```python
from build123d import *


# Read off the part's stored shape, not the designer's step: Shell1
with BuildPart() as part:
    # Sketch3 → Revolve1 (revolve)
    with BuildSketch(Plane(origin=(0, 0, 0), x_dir=(0, 0, -1), z_dir=(1, 0, 0)), mode=Mode.PRIVATE) as revolve1_sk:
        Polygon((-144.855352602, 25), (5.144647398, 25), (5.144647398, 22), (6.144647398, 22), (26.144647398, 20.250226729), (26.144647398, 0), (-144.855352602, 0), align=None)
    revolve(revolve1_sk.sketch.rotate(Axis((0, 0, 32.959641256), (0, 0, -1)), 90), axis=Axis((0, 0, 32.959641256), (0, 0, -1)))

    # Shell1 outline → Shell1 (revolve, cut)
    with BuildSketch(Plane.XZ):
        Polygon((19, -2.144647398), (22, -2.144647398), (22, 144.855352602), (0, 144.855352602), (0, -26.144647398), (17.238767217, -26.144647398), (19, -6.013664569), align=None)
    revolve(axis=Axis((0, 0, 0), (0, 0, 1)), mode=Mode.SUBTRACT)

    # Sketch4 → Revolve3 (revolve)
    with BuildSketch(Plane(origin=(0, 0, 0), x_dir=(0, 0, -1), z_dir=(1, 0, 0)), mode=Mode.PRIVATE) as revolve3_sk:
        with BuildLine():
            Line((-15.655352602, 37.557879022), (-15.655352602, 25))
            Line((-15.655352602, 25), (5.144647398, 25))
            Line((5.144647398, 25), (5.144647398, 37.557879022))
            Line((5.144647398, 37.557879022), (0.144647398, 37.557879022))
            ThreePointArc((0.144647398, 37.557879022), (-2.092417968, 32.142324694), (-2.855352602, 26.332796239))
            Line((-2.855352602, 26.332796239), (-7.655352602, 26.332796239))
            ThreePointArc((-7.655352602, 26.332796239), (-8.418287237, 32.142324694), (-10.655352602, 37.557879022))
            Line((-10.655352602, 37.557879022), (-15.655352602, 37.557879022))
        make_face()
    revolve(revolve3_sk.sketch.rotate(Axis((0, 0, -29.694647398), (0, 0, 1)), 90), axis=Axis((0, 0, -29.694647398), (0, 0, 1)))


solid = part.part
```
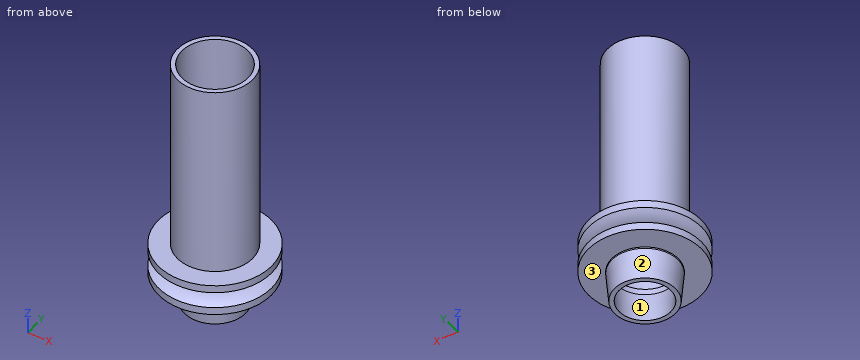
Here's how the part is built. I have some questions about the finished solid (model axes, mm). Face numbers are marked on the shaded views. Coordinates: 2 decimals unless noted, no trailing zeros. Write each loop counter-clockwise with the first axis right and the second up, starting at its lowest first coordinate (ties: lowest second). Pieces come first, ordered by that corner, then holes. Notation, with made-up numbers: (77, 43) -> (111, 43) arc R11 ccw to (111, 59) -> close; hole circle Ø10 at (10.5, 88.25). An arc over 180 degrees is marked (long way). Use a Markdown table: item, result. Add a question column.
(1) I'm going to push flat-ended pins straight in: P1, Ø5, axis at x = -13.5, z = 64.5, coming from the -Y side; P2, Ø12, axis at x = 8.5, z = 78, coming from the -Y side; P3, Ø10, axis at x = -4.5, z = 85.5, coming from the -Y side; P4, Ø22.5, axis at x = -11, y = 3.5, coming from the -Z side. Where does each tip first touch, or does it pass through?
(2) We'd pull the mould along Y, two halves only. Please class the marked faces 1, 2 and 3: +Y half, -Y half, draft (parallel to the pull), parting line (faces both ways), or undercut.
(3) If we section it at C-C, the plane z = 77.5: Write out the boundary of the cut face in (x, y), and give its area (3 significant figures).
(4) Please list where these lines run through material, in increasing order: line 1 (Z direction, x = -23, y = 14.5); line 2 (Y direction, x = 0, z = 72); line 3 (Y direction, x = 0, z = -3.75).
Outcome:
| question | item | result |
|---|---|---|
| 1 | P1 | stops at y = -22.45 |
| 1 | P2 | stops at y = -24.87 |
| 1 | P3 | stops at y = -25 |
| 1 | P4 | stops at z = -26.14 |
| 2 | face 1 | undercut |
| 2 | face 2 | parting line |
| 2 | face 3 | draft |
| 3 | outline | circle Ø50 at (0, 0); hole circle Ø44 at (0, 0) |
| 3 | area | 443 mm^2 |
| 4 | line 1 | z = -5.14 to 2.84, 7.67 to 15.66 |
| 4 | line 2 | y = -25 to -22, 22 to 25 |
| 4 | line 3 | y = -37.56 to -19, 19 to 37.56 |
